```python
from build123d import *

# Parameters (mm, degrees)
F0_W     = 121.572584
F0_H     = 86.733874
F1_DEPTH = 50
F2_R     = 18.878817
F3_DEPTH = 50
F4_SIZE  = 5
F5_R     = 5


with BuildPart() as f1:
    # F0 (on Top) → F1 (new body)
    with BuildSketch(Plane.XY):
        with Locations((1.088709, 3.084676)):
            Rectangle(F0_W, F0_H)
    extrude(amount=F1_DEPTH)

    # F2 (on face) → F3 (cut)
    with BuildSketch(Plane.XY.offset(50)):
        Circle(F2_R)
    extrude(amount=-F3_DEPTH, mode=Mode.SUBTRACT)

    # F4
    f4_edges = [f1.edges().sort_by_distance(p)[0] for p in [
        (1.088709, -40.282261, 50),
        (61.875001, 3.084676, 50),
        (1.088709, 46.451613, 50),
        (-59.697583, 3.084676, 50),
    ]]
    chamfer(f4_edges, length=F4_SIZE)

    # F5
    f5_edges = [f1.edges().sort_by_distance(p)[0] for p in [
        (61.875001, 3.084676, 0),
        (1.088709, -40.282261, 0),
        (-59.697583, 3.084676, 0),
        (1.088709, 46.451613, 0),
    ]]
    fillet(f5_edges, radius=F5_R)


solid = f1.part
```
Could you check a few things on this model? Use its own coordinates, in mm. Coordinates: 2 decimals unless noted, no trailing zeros. Order: outer loops, then holes, each group sorted by start corner. A loop starts at its lowest first (then second) coordinate and runs counter-clockwise, first axis right, second up. Notation, with made-up numbers: M 10.5,62.5 L 51.5,62.5 A20 ccw 51.5,66.5 Z; hole C 35,5.25 d5. An arc over 180 degrees is marked long. Use one line per item in the form item = value. Start each with the question number.
1. We'd pull the mould along X, two halves only. Please class faces 1 (the flat face through (-57.2, 2.5, 47.5)), 2 (the flat face through (59.41, 2.478, 47.465)), 3 (the cylindrical face through (18.007, 5.671, 25.35)), 4 (the flat face through (0, -40.282, 25)): +X half, -X half, draft (parallel to the pull), parting line (faces both ways), or undercut.
2. Please list where these lines run through material, in increasing order: line 1 (Y direction, x = 0, z = 23.5); line 2 (X direction, y = 10.5, z = 13) (3 decimals); line 3 (Y direction, x = -8, z = 28.5).
3. Suppose I cut it at A-A on x = 0. Write out the boundary of the cut face in (y, z), then the cut area to 3 significant figures.
4. Suppose I cut it at B-B on y = 0. Write out the boundary of the cut face in (x, z) (3 decimals).
5. Suppose I cut it at C-C on z = 38. Write out the boundary of the cut face in (x, y) (3 decimals).
6. For pin 1 (2 mm diameter, centred on x = -2, y = -17, fed in from +Z) (3 decimals), with a flat end and sliding along its axis, tell me the tip position at first contact or that it passes through.
Geometry says:
q1.face_1 = -X half
q1.face_2 = +X half
q1.face_3 = undercut
q1.face_4 = draft
q2.line_1 = -40.28 to -18.88, 18.88 to 46.45
q2.line_2 = -59.698 to -15.689, 15.689 to 61.875
q2.line_3 = -40.28 to -17.1, 17.1 to 46.45
q3.outline = M -40.28,5 A5 ccw -35.28,0 L -18.88,0 L -18.88,50 L -35.28,50 L -40.28,45 Z; M 18.88,0 L 41.45,0 A5 ccw 46.45,5 L 46.45,45 L 41.45,50 L 18.88,50 Z
q3.area = 2,410 mm^2
q4.outline = M -59.698,5 A5 ccw -54.698,0 L -18.879,0 L -18.879,50 L -54.698,50 L -59.698,45 Z; M 18.879,0 L 56.875,0 A5 ccw 61.875,5 L 61.875,45 L 56.875,50 L 18.879,50 Z
q5.outline = M -59.698,-40.282 L 61.875,-40.282 L 61.875,46.452 L -59.698,46.452 Z; hole C 0,0 d37.758
q6.pin_1 = through
